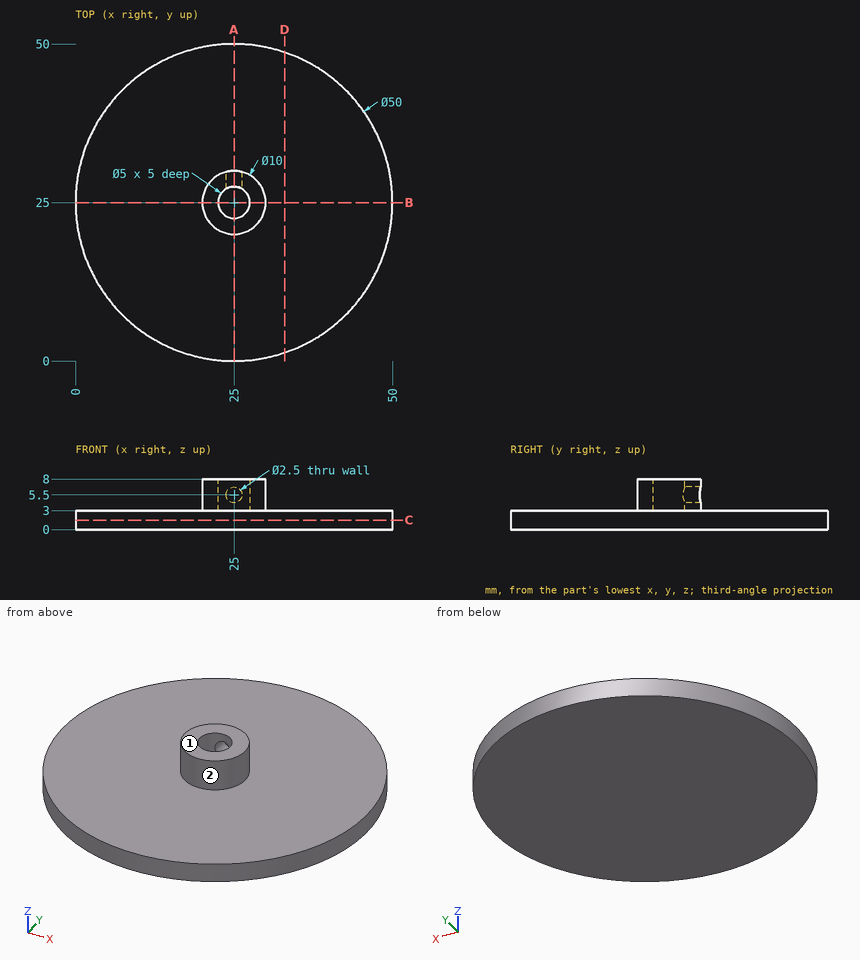
Geometry check sheet. Reference: drawing and pictorial views, mm from the part's lowest x, y, z. A direction names the side the tool comes from. Give positions to 0.01 mm unless a question says otherwise; leave off trailing zeros. Write each loop counter-clockwise with the first axis right and the second up, starting at its lowest first coordinate (ties: lowest second). Pieces come first, ordered by that corner, then holes. Notation, with made-up numbers: M 89.25,12.25 L 114.25,12.25 A23 cw 114.25,50.25 Z; hole C 60,-18.5 d11. An arc over 180 degrees is marked long. Put each result on its own line as item: value. Start each with the question number.
1. Section check D-D (x = 33). Record the cut outline in (y, z), and give its area (3 significant figures).
2. Section check B-B (y = 25). Record the cut outline in (x, z).
3. Go/stop test with flat-tipped pins: pin 1 Ø1.5 at (y, z) = (36.5, 3) entering from +X; pin 2 Ø3 at (x, z) = (25, 5.5) entering from +Y; pin 3 Ø4.5 at (x, y) = (25, 25) entering from +Z. Record where each tip stops, or that it passes through.
4. Scan lines: line 1 along Z through (x, y) = (25, 28); line 2 along Z through (x, y) = (33, 13.5); line 3 along Y through (x, z) = (25, 4.7). Record each from-to range of solid material in increasing order. Write a range as [from, to].
5. Section check A-A (x = 25). Record the cut outline in (y, z), and give its area (3 significant figures).
6. Section check C-C (z = 1.5). Record the cut outline in (x, y).
7. Set-up check for the marked faces 1 and 2: record each of +Z, -Z, +X, -X, +Y, -Y from which the full face is reachable in a straight line by a thin tool's end or side.
Answer list:
1. outline: M 1.31,0 L 48.69,0 L 48.69,3 L 1.31,3 Z
1. area: 142 mm2
2. outline: M 0,0 L 50,0 L 50,3 L 30,3 L 30,8 L 27.5,8 L 27.5,3 L 22.5,3 L 22.5,8 L 20,8 L 20,3 L 0,3 Z
3. pin 1: x = 47.57
3. pin 2: y = 30
3. pin 3: z = 3
4. line 1: [0, 4.25], [6.75, 8]
4. line 2: [0, 3]
4. line 3: [20, 22.5]
5. outline: M 0,0 L 50,0 L 50,3 L 30,3 L 30,4.25 L 27.5,4.25 L 27.5,3 L 22.5,3 L 22.5,8 L 20,8 L 20,3 L 0,3 Z; M 27.5,6.75 L 30,6.75 L 30,8 L 27.5,8 Z
5. area: 169 mm2
6. outline: C 25,25 d50
7. face 1: +Z, +X, -X, +Y, -Y
7. face 2: +Z
